The listing builds one solid part. Answer for the finished solid, in the listing's coordinates (mm). A direction names the side the tool comes from. Give positions to 0.01 mm unless a question says otherwise; leave off trailing zeros. Order: outer loops, then holes, each group sorted by start corner. A loop starts at its lowest first (then second) coordinate and runs counter-clockwise, first axis right, second up. Notation, with made-up numbers: (-18, 87) - (35, 87) arc R15 ccw to (35, 95) - close; hole circle Ø6 at (44.5, -24.5). An arc over 180 degrees is marked (long way). Use a Markdown table: item, result. Add a question column.
1) Straight lines are drawn through the part: line 1 (Y direction, x = 40, z = -16); line 2 (X direction, y = 2, z = -19); line 3 (Z direction, x = 33, y = 30.5). For each, find the intervals that lie inside material, in ascending order.
2) For faces 4 (the face through (47, 16, -20.2)), 5 (the face through (-29.97, 2.46, -1.32)), 6 (the face through (32.5, 18, -18)), 7 (the face through (46.1, 16, -18)), 8 (the face through (47, 16, -15.2)), determine the directions among +Z, -Z, +X, -X, +Y, -Y from which every point of the face is accessible in a straight line to the end or side of a thin tool.
3) Find section B-B, the plane x = 38. Determine the outline of the cut face in (y, z).
4) Find section C-C, the plane y = 29.7. Determine the outline of the cut face in (x, z), plus the area to 3 significant figures.
5) Find section A-A, the plane y = 2.3. Determine the outline of the cut face in (x, z).
6) Flat-ended cylindrical pins translate along their axes: pin 1 (5 mm diameter, centred on x = 30.5, y = 10.5, fed in from -Z); pin 2 (1.6 mm diameter, centred on x = 40, y = 2.3, fed in from -Z); pin 3 (5.5 mm diameter, centred on x = 29, y = 3.5, fed in from -Z); pin 4 (2.5 mm diameter, centred on y = 3.5, z = -24, fed in from +X). Find the tip coordinate at first contact, or state that the pin passes through.
7) The mould has two halves that part along Y. Classify faces 1 (the face through (40.954, 2.6, -17.735)), 2 (the face through (40, 32, -18)), 3 (the face through (47.5, 16, -18)): released by +Y, released by -Y, zero draft, split by the parting line, or undercut.
from build123d import *

# Parameters (mm, degrees)
SKETCH1_R           = 30
BOSS_EXTRUDE1_DEPTH = 5
BOSS_EXTRUDE4_START = -20.2
SKETCH3_W           = 15
SKETCH3_H           = 32
SKETCH3_R           = 1
SKETCH3_W_2         = 12.2
SKETCH3_H_2         = 22.8
BOSS_EXTRUDE4_DEPTH = 5


with BuildPart() as part:
    # Sketch1 → Boss-Extrude1 (new body)
    with BuildSketch(Plane(origin=(0, 0, 0), x_dir=(1, 0, 0), z_dir=(0, 1, 0))):
        with BuildLine():
            Line((32.5, 0), (32.5, 26))
            Line((32.5, 26), (19.5, 26))
            ThreePointArc((19.5, 26), (-29.068883707, -14.534441854), (32.5, 0))
        make_face()
        Circle(SKETCH1_R, mode=Mode.SUBTRACT)
    extrude(amount=BOSS_EXTRUDE1_DEPTH)

    # Sketch3 → Boss-Extrude4 (add)
    with BuildSketch(Plane.XY.offset(BOSS_EXTRUDE4_START)):
        with Locations((40, 16)):
            Rectangle(SKETCH3_W, SKETCH3_H)
        with Locations((40, 29.7)):
            Circle(SKETCH3_R, mode=Mode.SUBTRACT)
        with Locations((40, 2.3)):
            Circle(SKETCH3_R, mode=Mode.SUBTRACT)
        with Locations((40, 16)):
            Rectangle(SKETCH3_W_2, SKETCH3_H_2, mode=Mode.SUBTRACT)
    extrude(amount=BOSS_EXTRUDE4_DEPTH)


solid = part.part
The answers:
| question | item | result |
|---|---|---|
| 1 | line 1 | 0 to 1.3, 3.3 to 4.6, 27.4 to 28.7, 30.7 to 32 |
| 1 | line 2 | -26.37 to -23.22, 23.22 to 39.05, 40.95 to 47.5 |
| 1 | line 3 | -20.2 to -15.2 |
| 2 | face 4 | -Z, +X, +Y, -Y |
| 2 | face 5 | +Y, -Y |
| 2 | face 6 | +Z, -Z, -X, +Y |
| 2 | face 7 | +Z, -Z |
| 2 | face 8 | +Z, +X, +Y, -Y |
| 3 | outline | (0, -20.2) - (4.6, -20.2) - (4.6, -15.2) - (0, -15.2) - close; (27.4, -20.2) - (32, -20.2) - (32, -15.2) - (27.4, -15.2) - close |
| 4 | outline | (32.5, -20.2) - (39, -20.2) - (39, -15.2) - (32.5, -15.2) - close; (41, -20.2) - (47.5, -20.2) - (47.5, -15.2) - (41, -15.2) - close |
| 4 | area | 65.0 mm2 |
| 5 | outline | (19.5, -26) - (32.5, -26) - (32.5, -20.2) - (39, -20.2) - (39, -15.2) - (32.5, -15.2) - (32.5, 0) arc R32.5 ccw (long way) to start; (41, -20.2) - (47.5, -20.2) - (47.5, -15.2) - (41, -15.2) - close; hole circle Ø60 at (0, 0) |
| 6 | pin 1 | z = -20.2 |
| 6 | pin 2 | through |
| 6 | pin 3 | z = -26 |
| 6 | pin 4 | x = 32.5 |
| 7 | face 1 | undercut |
| 7 | face 2 | released by +Y |
| 7 | face 3 | zero draft |
